Read the model definition and answer for the solid it produces. Units are mm, in the model's axes. A direction names the side the tool comes from. Round coordinates to 2 decimals unless told otherwise and drop trailing zeros. Order: outer loops, then holes, each group sorted by start corner. A loop starts at its lowest first (then second) coordinate and runs counter-clockwise, first axis right, second up. Notation, with made-up numbers: M 74,80.25 L 97,80.25 A14 cw 97,84.25 Z; hole C 25.5,17.5 d10. An arc over 180 degrees is marked long. Answer as CSV lines item,"result".
```python
from build123d import *

# Parameters (mm, degrees)
F0_R       = 14.1
F1_DEPTH   = 16
F2_SIZE    = 1
F3_R       = 5.7
F4_DEPTH   = 8
F5_R       = 6.7
F5_R_2     = 5.7
F6_DEPTH   = 4
F7_SIZE2   = 2
F7_SIZE    = 1
F7_2_SIZE2 = 1.99999
F7_2_SIZE  = 0.99999
F8_W       = 13.4
F8_H       = 6
F9_DEPTH   = 10


# Not quite as in the source:
# - a fillet or chamfer is up to 0.001 mm smaller than in the source, because OpenCascade refuses the exact size


with BuildPart() as f1:
    # F0 (on Top) → F1 (new body)
    with BuildSketch(Plane.XY):
        Circle(F0_R)
        with BuildLine():
            Line((-12.0586068847, -1), (-5.7131427428, -1))
            ThreePointArc((-5.7131427428, -1), (-4.1012193309, -4.1012193309), (-1, -5.7131427428))
            Line((-1, -5.7131427428), (-1, -12.0586068847))
            ThreePointArc((-1, -12.0586068847), (-8.5559920524, -8.5559920524), (-12.0586068847, -1))
        make_face(mode=Mode.SUBTRACT)
        with BuildLine():
            ThreePointArc((12.0586068847, -1), (8.5559920524, -8.5559920524), (1, -12.0586068847))
            Line((1, -12.0586068847), (1, -5.7131427428))
            ThreePointArc((1, -5.7131427428), (4.1012193309, -4.1012193309), (5.7131427428, -1))
            Line((5.7131427428, -1), (12.0586068847, -1))
        make_face(mode=Mode.SUBTRACT)
        with BuildLine():
            ThreePointArc((-12.0586068847, 1), (-8.5559920524, 8.5559920524), (-1, 12.0586068847))
            Line((-1, 12.0586068847), (-1, 5.7131427428))
            ThreePointArc((-1, 5.7131427428), (-4.1012193309, 4.1012193309), (-5.7131427428, 1))
            Line((-5.7131427428, 1), (-12.0586068847, 1))
        make_face(mode=Mode.SUBTRACT)
        with BuildLine():
            Line((12.0586068847, 1), (5.7131427428, 1))
            ThreePointArc((5.7131427428, 1), (4.1012193309, 4.1012193309), (1, 5.7131427428))
            Line((1, 5.7131427428), (1, 12.0586068847))
            ThreePointArc((1, 12.0586068847), (8.5559920524, 8.5559920524), (12.0586068847, 1))
        make_face(mode=Mode.SUBTRACT)
    extrude(amount=F1_DEPTH)

    # F2
    f2_edges = [f1.edges().sort_by_distance(p)[0] for p in [
        (-14.1, 0, 0),
    ]]
    chamfer(f2_edges, length=F2_SIZE)

    # F3 (on face) → F4 (join)
    with BuildSketch(Plane.XY.offset(16)):
        Circle(F3_R)
    extrude(amount=F4_DEPTH)

    # F5 (on face) → F6 (join)
    with BuildSketch(Plane.XY.offset(24)):
        Circle(F5_R)
        Circle(F5_R_2, mode=Mode.SUBTRACT)
    extrude(amount=-F6_DEPTH)

    # F7
    f7_edges = [f1.edges().sort_by_distance(p)[0] for p in [
        (-6.7, 0, 24),
    ]]
    f7_side = f1.faces().sort_by_distance((0, 0, 24))[0]
    chamfer(f7_edges, length=F7_SIZE, length2=F7_SIZE2, reference=f7_side)

    # F7#2 (size 1 and 2 in the source; OpenCascade refuses exactly that, so slightly less here)
    f7_2_edges = [f1.edges().sort_by_distance(p)[0] for p in [
        (-6.7, 0, 20),
    ]]
    f7_2_side = f1.faces().sort_by_distance((-6.510495, 0, 20))[0]
    chamfer(f7_2_edges, length=F7_2_SIZE, length2=F7_2_SIZE2, reference=f7_2_side)

    # F8 (on face) → F9 (cut)
    with BuildSketch(Plane.XY.offset(24)):
        Rectangle(F8_W, F8_H)
    extrude(amount=-F9_DEPTH, mode=Mode.SUBTRACT)


solid = f1.part
```
Item 1: A cutting plane is placed at A-A, the plane z = 11.5. Determine the outline of the cut face in (x, y), and give its area (3 significant figures).
Ans:
outline,"C 0,0 d28.2; hole M -12.06,-1 A12.1 ccw -1,-12.06 L -1,-5.71 A5.8 cw -5.71,-1 Z; hole M -12.06,1 L -5.71,1 A5.8 cw -1,5.71 L -1,12.06 A12.1 ccw Z; hole M 1,-12.06 A12.1 ccw 12.06,-1 L 5.71,-1 A5.8 cw 1,-5.71 Z; hole M 1,5.71 A5.8 cw 5.71,1 L 12.06,1 A12.1 ccw 1,12.06 Z"
area,"321 mm2"
Item 2: Flat-ended cylindrical pins translate along their axes: pin 1 (12 mm diameter, centred on x = 5, z = 15.5, fed in from +Y); pin 2 (8 mm diameter, centred on x = -10, z = 2.5, fed in from +Y); pin 3 (8 mm diameter, centred on x = -5, z = 17.5, fed in from +Y); pin 4 (5 mm diameter, centred on y = -9.5, z = 11, fed in from -X). Find the tip coordinate at first contact, or state that the pin passes through.
Ans:
pin 1,"y = 14.1"
pin 2,"y = 12.76"
pin 3,"y = 14.04"
pin 4,"x = -12.24"
Item 3: Find the intervals of material crossed by probe 1 along X at (y, z) = (8, 7.75); probe 2 along X at (y, z) = (7, 3); probe 3 along Y at (x, z) = (4, 3.75), in increasing order. Write a range as [from, to].
Ans:
probe 1,"[-11.61, -9.08], [-1, 1], [9.08, 11.61]"
probe 2,"[-12.24, -9.87], [-1, 1], [9.87, 12.24]"
probe 3,"[-13.52, -11.42], [-4.2, 4.2], [11.42, 13.52]"
Item 4: A tool of negligible diameter and unlimited length cuts with its end or side. For faces 4 (the face through (-6.7, 0, 15)), 5 (the face through (4.1, -4.1, 7.9)), 6 (the face through (-9, 1, 8)), from which of +Z, -Z, +X, -X, +Y, -Y can it reach the whole face along a straight path? Write none if from no direction.
Ans:
face 4,"+Z"
face 5,"-Z"
face 6,"+Z, -Z"
Item 5: A cutting plane is placed at B-B, the plane y = 0. Determine the outline of the cut face in (x, z), and give its area (3 significant figures).
Ans:
outline,"M -14.1,1 L -13.1,0 L 13.1,0 L 14.1,1 L 14.1,16 L 6.7,16 L 6.7,14 L -6.7,14 L -6.7,16 L -14.1,16 Z"
area,"423 mm2"
Item 6: Determine the mould class of faces 1 (the face through (0, 3, 19)), 2 (the face through (0.1, 6, 20.6)), 3 (the face through (0, 0, 0)) for opening direction Z: +Z half, -Z half, draft (parallel to the pull), parting line (faces both ways), or undercut.
Ans:
face 1,"draft"
face 2,"undercut"
face 3,"-Z half"
Item 7: A cutting plane is placed at C-C, the plane z = 14.5. Determine the outline of the cut face in (x, y), and give its area (3 significant figures).
Ans:
outline,"C 0,0 d28.2; hole M -12.06,-1 A12.1 ccw -1,-12.06 L -1,-5.71 A5.8 cw -4.96,-3 L 4.96,-3 A5.8 cw 1,-5.71 L 1,-12.06 A12.1 ccw 12.06,-1 L 6.7,-1 L 6.7,1 L 12.06,1 A12.1 ccw 1,12.06 L 1,5.71 A5.8 cw 4.96,3 L -4.96,3 A5.8 cw -1,5.71 L -1,12.06 A12.1 ccw -12.06,1 L -6.7,1 L -6.7,-1 Z"
area,"251 mm2"
Item 8: A cutting plane is placed at D-D, the plane x = -2. Give the number of separate pieces and of enclosed holes in the cut face, and give its area (3 significant figures).
Ans:
separate pieces,"3"
enclosed holes,"0"
area,"268 mm2"
